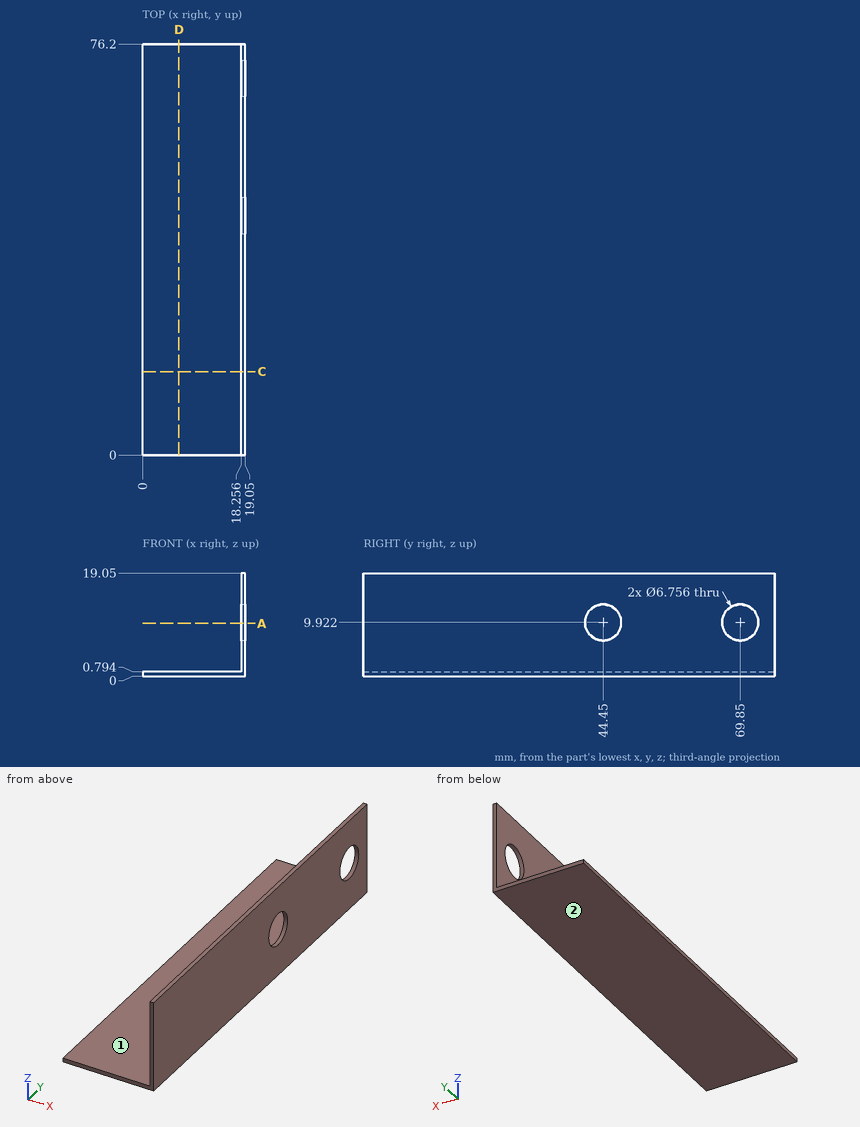
Geometry check sheet. Reference: drawing and pictorial views, mm from the part's lowest x, y, z. A direction names the side the tool comes from. Round coordinates to 2 decimals unless told otherwise and drop trailing zeros. Loops run counter-clockwise (first coordinate to the right, second up) from the corner with the lowest first, then second, coordinate; pieces in that order, holes last. Notation, with made-up numbers: (-4.5, -29) - (16.5, -29) arc R13 cw to (16.5, -24) - close; hole circle Ø11 at (1.5, 9.25). An arc over 180 degrees is marked (long way). Answer in a Markdown table with one row per item. Add a question column.
Q1. Section check C-C on y = 15.5. Enter the section's corners in (x, z).
Q2. Gauge pin test, flat ends, axial feed: pin 1 (9 mm diameter, centred on x = 8, y = 50, fed in from +Z); pin 2 (4 mm diameter, centred on y = 69.85, z = 9.92, fed in from -X); pin 3 (1 mm diameter, centred on y = 29.5, z = 10, fed in from -X). Record the tip position at first contact, or that the pin passes through.
Q3. Section check D-D on x = 6.75. Enter the section's corners in (y, z).
Q4. Material ranges on line 1 (Z direction, x = 18.55, y = 69.85); line 2 (Z direction, x = 2.5, y = 50); line 3 (X direction, y = 17.5, z = 2), recorded low to high.
Q5. Tool access check on the marked faces 1 and 2. Record the directions out of +Z, -Z, +X, -X, +Y, -Y that give a thin tool (end or side, any length) a straight path to the whole face; none if there is none.
Q6. Section check A-A on z = 9.75. Enter the section's corners in (x, y).
Found:
| question | item | result |
|---|---|---|
| 1 | outline | (0, 0) - (19.05, 0) - (19.05, 19.05) - (18.26, 19.05) - (18.26, 0.79) - (0, 0.79) - close |
| 2 | pin 1 | stops at z = 0.79 |
| 2 | pin 2 | passes through |
| 2 | pin 3 | stops at x = 18.26 |
| 3 | outline | (0, 0) - (76.2, 0) - (76.2, 0.79) - (0, 0.79) - close |
| 4 | line 1 | z = 0 to 6.54, 13.3 to 19.05 |
| 4 | line 2 | z = 0 to 0.79 |
| 4 | line 3 | x = 18.26 to 19.05 |
| 5 | face 1 | +Z, -X, +Y, -Y |
| 5 | face 2 | -Z, +X, -X, +Y, -Y |
| 6 | outline | (18.26, 0) - (19.05, 0) - (19.05, 41.08) - (18.26, 41.08) - close; (18.26, 47.82) - (19.05, 47.82) - (19.05, 66.48) - (18.26, 66.48) - close; (18.26, 73.22) - (19.05, 73.22) - (19.05, 76.2) - (18.26, 76.2) - close |
